Geometry check sheet. Reference: the model listing, model coordinates, mm. A direction names the side the tool comes from. Round coordinates to 2 decimals unless told otherwise and drop trailing zeros. Write each loop counter-clockwise with the first axis right and the second up, starting at its lowest first coordinate (ties: lowest second). Pieces come first, ordered by that corner, then holes.
Item 1: Scan lines: probe 1 along Y at (x, z) = (21, -15) (1 decimal); probe 2 along Z at (x, y) = (21, 23); probe 3 along Y at (x, z) = (2, -46). Record each from-to range of solid material in increasing order.
Item 2: Cross-section at B-B (z = -57.5). Enter the section's corners in (x, y), then the cut area to 3 significant figures.
Item 3: Cross-section at D-D (z = -15). State how many separate pieces and enclosed holes the cut face has, then the cut area to 3 significant figures.
Item 4: Cross-section at A-A (y = 15.06). Enter the section's corners in (x, z) (3 decimals).
Item 5: Draft check along Z on faces 5 (the face through (15, 28, 0)), 6 (the face through (14.865, 104.88, -14.16)), 7 (the face through (25.995, 7.502, -17.272)). Enter one of: pulls with the +Z half, pulls with the -Z half, needs draft (parallel to the pull), parting line crosses it, or undercut.
Item 6: Access from +Z, -Z, +X, -X, +Y, -Y to the whole of each face (thin tool, end or side, straight path). Record for faces 1 (the face through (3.042, 173.046, -14.16)), 2 (the face through (22.1, 4.5, -13)), 3 (the face through (15, 55.293, 22)), 4 (the face through (10, 16, -25.05)).
Item 7: Cross-section at C-C (x = 28). Enter the section's corners in (y, z) (3 decimals).
Item 8: Depth check by flat-ended pin: P1, Ø8, axis at y = 6.56, z = -15, coming from the -X side; P2, Ø4, axis at x = 21, z = -26.5, coming from the -Y side; P3, Ø9, axis at x = 12.5, y = 19, coming from the -Z side; P4, Ø3, axis at y = 15.06, z = -15, coming from the +X side. Enter the tip coordinate at first touch or a pass-through.
Autodesk Inventor part; units mm, degrees
ref_plane "Work Plane1" through (0, 0, -15) normal (0, 0, 1) x (1, 0, 0)
ref_plane "YZ Plane" through (0, 0, 0) normal (1, 0, 0) x (0, 1, 0)
ref_plane "XZ Plane" through (0, 0, 0) normal (0, 1, 0) x (-1, 0, 0)
sketch "Sketch1" plane through (0, 0, 0) normal (0, 0, 1) x (1, 0, 0)
  line L0 (0, 0) -> (25, 0)
  line L1 (25, 0) -> (25, 40)
  line L2 (25, 40) -> (0, 40)
  line L3 (0, 40) -> (0, 0)
  dimension "d1" = 25
  dimension "d2" = 40
  dimension "d3" = 25
extrude "Extrusion1" add sketch "Sketch1" against normal blind 30
sketch "Sketch2" plane through (25, 0, 0) normal (1, 0, 0) x (0, 0, -1)
  line L0 (0, 0) -> (30, 0)
  circle A0 centre (15, 6.56) radius 2.46
extrude "Extrusion2" cut sketch "Sketch2" against normal blind 30
sketch "Sketch3" plane through (0, 0, 0) normal (-1, 0, 0) x (0, 0, 1)
  line L0 (0, 0) -> (-30, 0)
  line L1 (-25.05, 0) -> (-4.95, 0)
  line L2 (-4.95, 0) -> (-4.95, 33.12)
  line L3 (-4.95, 33.12) -> (-25.05, 33.12)
  line L4 (-25.05, 33.12) -> (-25.05, 0)
  dimension "d11" = 20.1
extrude "Extrusion3" cut sketch "Sketch3" against normal blind 20
sketch "Sketch4" plane through (0, 0, 0) normal (0, -1, 0) x (1, 0, 0)
  line L0 (20, -4.95) -> (20, -25.05)
  line L1 (20, -15) -> (25, -15)
  line L2 (25, 0) -> (25, -30)
  line L3 (20, -8.025) -> (25, -8.025)
  line L4 (25, -8.025) -> (25, -21.975)
  line L5 (25, -21.975) -> (20, -21.975)
  line L6 (20, -21.975) -> (20, -8.025)
  line L7 (20, -8.025) -> (25, -21.975) construction
  line L8 (25, -8.025) -> (20, -21.975) construction
  line L9 (25, -12.54) -> (25, -17.46)
  point P0 (0, 0)
  point P1 (22.5, -15)
  dimension "d14" = 13.95
extrude "Extrusion4" add sketch "Sketch4" along normal blind 15
sketch "Sketch5" plane through (20, 0, 0) normal (-1, 0, 0) x (0, 0, 1)
  circle A0 centre (-15, 6.56) radius 2.46
  circle A1 centre (-15, 6.56) radius 4.7025
  circle A2 centre (-15, 6.56) radius 2.46
  circle A3 centre (-15, 6.56) radius 2.46
  point P0 (0, 0)
  dimension "d17" = 9.405
extrude "Extrusion5" cut sketch "Sketch5" against normal blind 2.1
sketch "Sketch6" plane through (25, 0, 0) normal (1, 0, 0) x (0, 0, -1)
  circle A0 centre (15, 6.56) radius 4.7025
  line L0 (15, 6.56) -> (15, 23.56)
  circle A1 centre (15, 23.56) radius 2.46
  point P0 (0, 0)
  dimension "d20" = 17
  dimension "d21" = 4.92
extrude "Extrusion6" cut sketch "Sketch6" against normal blind 10 contours A1
sketch "Sketch7" plane through (20, 0, 0) normal (-1, 0, 0) x (0, 0, 1)
  circle A0 centre (-15, 23.56) radius 2.46
  circle A1 centre (-15, 23.56) radius 4.7025
  point P0 (0, 0)
  dimension "d24" = 9.405
extrude "Extrusion7" cut sketch "Sketch7" against normal blind 2.1
sketch "Sketch9" plane through (25, 0, 0) normal (1, 0, 0) x (0, 0, -1)
  circle A0 centre (15, 6.56) radius 2.46
  circle A1 centre (15, 6.56) radius 2.46
  circle A2 centre (15, 23.56) radius 2.46
  circle A3 centre (15, 23.56) radius 2.46
  line L0 (30, 40) -> (30, 0)
  line L1 (30, 0) -> (30, 40)
  line L2 (30, 40) -> (0, 40)
  line L3 (0, 40) -> (0, 0)
  line L4 (0, 0) -> (8.025, 0)
  line L5 (21.975, 0) -> (21.975, -15)
  line L6 (21.975, -15) -> (8.025, -15)
  line L7 (8.025, -15) -> (8.025, 0)
  line L8 (0, 0) -> (8.025, 0)
  line L9 (21.975, 0) -> (30, 0)
extrude "Extrusion8" add sketch "Sketch9" along normal blind 5
sketch "Sketch10" plane through (0, 40, 0) normal (0, 1, 0) x (1, 0, 0)
  line L0 (0, 30) -> (30, 30)
  line L1 (30, 0) -> (0, 0)
  line L2 (0, 30) -> (30, 30)
  line L3 (30, 30) -> (30, 0)
  line L4 (30, 0) -> (0, 0)
  line L5 (0, 0) -> (0, 30)
extrude "Extrusion9" add sketch "Sketch10" along normal blind 30
sketch "Sketch12" plane through (30, 0, 0) normal (1, 0, 0) x (0, 0, -1)
  circle A0 centre (15, 6.56) radius 2.46
  line L0 (15, 6.56) -> (15, 15.06)
  circle A1 centre (15, 15.06) radius 2.525
  point P0 (0, 0)
  dimension "d31" = 8.5
  dimension "d33" = 5.05
extrude "Extrusion10" cut sketch "Sketch12" against normal blind 30 contours A1
sketch "Sketch15" plane through (0, 0, -25.05) normal (-1, 0, 0) x (0, 0, 1)
  line L0 (0, 33.12) -> (20.1, 33.12)
  line L1 (20.1, 33.12) -> (20.1, 0)
  line L2 (0, 33.12) -> (20.1, 33.12)
  line L3 (20.1, 33.12) -> (20.1, 31.1)
  line L4 (20.1, 31.1) -> (0, 31.1)
  line L5 (0, 31.1) -> (0, 33.12)
  point P0 (25.05, 0)
  dimension "d57" = 2.02
extrude "Extrusion13" add sketch "Sketch15" against normal blind 20
sketch "Sketch17" plane through (0, 0, 0) normal (0, 0, 1) x (1, 0, 0)
  line L0 (0, 70) -> (30, 70)
  line L1 (30, 70) -> (50.0622, 90.0622)
  line L2 (30, 70) -> (80, 70) construction
  line L3 (11.9522, 97.2454) -> (0, 85.2932)
  line L4 (0, 70) -> (0, 85.2932)
  line L5 (0, 70) -> (0, 0)
  line L6 (0, 70) -> (30, 70)
  line L7 (10.923, 112.2849) -> (0, 120.567)
  line L8 (50.0622, 105.3553) -> (50.0622, 120.567)
  line L9 (50.0622, 105.3553) -> (50.0622, 90.0622)
  arc A0 (11.9522, 97.2454) -> (10.923, 112.2849) centre (4.8811, 104.3165) ccw
  line L10 (0, 174.567) -> (30, 174.567)
  line L11 (30, 174.567) -> (50.0622, 120.567)
  line L12 (6, 171.567) -> (0, 174.567)
  line L13 (6, 123.567) -> (0, 120.567)
  line L14 (6, 123.567) -> (12, 147.567)
  line L15 (6, 171.567) -> (12, 147.567)
  dimension "d61" = 45
  dimension "d62" = 32.0271
  dimension "d72" = 10
extrude "Extrusion14" add sketch "Sketch17" against normal blind 30
sketch "Sketch24" plane through (0, 0, 0) normal (0, 0, 1) x (1, 0, 0)
  line L0 (30, 70) -> (50.0622, 90.0622)
  line L1 (30, 70) -> (50.0622, 90.0622)
  line L2 (50.0622, 90.0622) -> (50.0622, 120.567)
  line L3 (50.0622, 90.0622) -> (50.0622, 120.567)
  line L4 (30, 174.567) -> (50.0622, 120.567)
  line L5 (50.0622, 120.567) -> (30, 174.567)
  line L6 (30, 174.567) -> (0, 174.567)
  line L7 (30, 174.567) -> (0, 174.567)
  line L8 (0, 174.567) -> (6, 171.567)
  line L9 (0, 174.567) -> (6, 171.567)
  line L10 (12, 147.567) -> (6, 171.567)
  line L11 (6, 171.567) -> (12, 147.567)
  line L12 (12, 147.567) -> (6, 123.567)
  line L13 (12, 147.567) -> (6, 123.567)
  line L14 (6, 123.567) -> (0, 120.567)
  line L15 (6, 123.567) -> (0, 120.567)
  line L16 (0, 120.567) -> (10.923, 112.2849)
  line L17 (0, 120.567) -> (10.923, 112.2849)
  line L18 (0, 85.2932) -> (11.9522, 97.2454)
  line L19 (11.9522, 97.2454) -> (0, 85.2932)
  line L20 (0, 85.2932) -> (0, 55.2932)
  line L21 (0, 0) -> (0, 85.2932)
  line L22 (0, 55.2932) -> (30, 55.2932)
  line L23 (30, 0) -> (30, 70)
  line L24 (30, 55.2932) -> (30, 70)
  arc A0 (11.9522, 97.2454) -> (10.923, 112.2849) centre (4.8811, 104.3165) ccw
  dimension "d106" = 30
extrude "Extrusion15" add sketch "Sketch24" along normal blind 45
ref_plane "Work Plane1" through (0, 0, -15) normal (0, 0, 1) x (1, 0, 0)
mirror "Mirror1" about plane through (0, 0, -15) normal (0, 0, 1) of "Extrusion15"
properties part number "rec_c_48mm_x_120mm"
Resolved:
1. probe 1: y = -15 to 1.9, 11.3 to 12.5, 17.6 to 18.9, 28.3 to 174.6
1. probe 2: z = -30 to -19.67, -10.33 to 0
1. probe 3: y = 55.29 to 87.29, 119.05 to 121.57, 173.57 to 174.57
2. outline: (0, 55.29) - (30, 55.29) - (30, 70) - (50.06, 90.06) - (50.06, 120.57) - (30, 174.57) - (0, 174.57) - (6, 171.57) - (12, 147.57) - (6, 123.57) - (0, 120.57) - (10.92, 112.28) arc R10 cw to (11.95, 97.25) - (0, 85.29) - close
2. area: 4,160 mm2
3. separate pieces: 4
3. enclosed holes: 0
3. area: 5,180 mm2
4. outline: (0, -30) - (30, -30) - (30, -17.525) - (20, -17.525) - (20, -25.05) - (0, -25.05) - close; (0, -4.95) - (20, -4.95) - (20, -12.475) - (30, -12.475) - (30, 0) - (0, 0) - close
5. face 5: pulls with the +Z half
5. face 6: needs draft
5. face 7: undercut
6. face 1: +Z, -Z, -X
6. face 2: -X
6. face 3: +Z, +X, -X, -Y
6. face 4: -X, -Y
7. outline: (-15, -21.975) - (0, -21.975) - (0, -30) - (55.293, -30) - (55.293, -75) - (174.567, -75) - (174.567, 45) - (55.293, 45) - (55.293, 0) - (0, 0) - (0, -8.025) - (-15, -8.025) - close; hole circle Ø4.92 at (6.56, -15); hole circle Ø5.05 at (15.06, -15); hole circle Ø4.92 at (23.56, -15)
8. P1: stops at x = 22.1
8. P2: stops at y = 0
8. P3: stops at z = -30
8. P4: passes through
